The listing builds one solid part. Answer for the finished solid, in the listing's coordinates (mm). Give positions to 0.01 mm unless a question says otherwise; leave off trailing zeros. Write each loop counter-clockwise with the first axis right and the second up, starting at its lowest first coordinate (ties: lowest second). Pieces come first, ordered by that corner, then holes. Notation, with made-up numbers: (-3, 60.5) - (10, 60.5) arc R31 ccw to (10, 93.5) - close; hole circle Ø8 at (44.25, -38.5). An arc over 180 degrees is marked (long way). Answer as CSV lines item,"result". Start each with the question number.
(1) Straight lines are drawn through the part: probe 1 along X at (y, z) = (1.25, -38); probe 2 along Z at (x, y) = (10, 3.8); probe 3 along Z at (x, y) = (27.25, 2.7). For each, find the intervals that lie inside material, in ascending order.
(2) Find section A-A (x = 27.25). Write down the section's boundary in (y, z), then the cut area to 3 significant figures.
(3) Find section D-D (y = 3.5). State how many separate pieces and enclosed holes the cut face has, then the cut area to 3 significant figures.
(4) For a pull along X with two mould halves and no side action, classify faces 1 (the face through (25, 0, -51)), 2 (the face through (46.91, 2.35, -37.63)), 3 (the face through (50, 2, -49)), 4 (the face through (0, 2, -51)) as pulls with the +X half, pulls with the -X half, needs draft (parallel to the pull), parting line crosses it, or undercut.
(5) Find section B-B (z = -66.6). Write down the section's boundary in (x, y).
(6) Find section C-C (z = -38). Write down the section's boundary in (x, y).
(7) This flat-tipped pin is pushed along its axis until it touches: pin 1 Ø2 at (x, z) = (36.5, -34) entering from -Y. Where does it stop, or does it pass through?
from build123d import *

# Parameters (mm, degrees)
SKETCH1_R           = 1.7
BOSS_EXTRUDE1_DEPTH = 4.7625


with BuildPart() as part:
    # Sketch1 → Boss-Extrude1 (new body)
    with BuildSketch(Plane(origin=(0, 0, 0), x_dir=(1, 0, 0), z_dir=(0, 1, 0))):
        Polygon((0, 90), (0, 10), (20, 10), (50, 10), (50, 90), align=None)
        with Locations(Location((10, 20, 0), (0, 0, 90))):
            Circle(SKETCH1_R, mode=Mode.SUBTRACT)
        with Locations(Location((27.25, 38, 0), (0, 0, 90))):
            Circle(SKETCH1_R, mode=Mode.SUBTRACT)
        with Locations(Location((45.25, 23, 0), (0, 0, 90))):
            Circle(SKETCH1_R, mode=Mode.SUBTRACT)
        with Locations(Location((45.25, 38, 0), (0, 0, 90))):
            Circle(SKETCH1_R, mode=Mode.SUBTRACT)
        with Locations(Location((10, 70, 0), (0, 0, 90))):
            Circle(SKETCH1_R, mode=Mode.SUBTRACT)
        with Locations(Location((45.25, 66.6, 0), (0, 0, 90))):
            Circle(SKETCH1_R, mode=Mode.SUBTRACT)
        with Locations(Location((27.25, 81.6, 0), (0, 0, 90))):
            Circle(SKETCH1_R, mode=Mode.SUBTRACT)
        with Locations(Location((45.25, 81.6, 0), (0, 0, 90))):
            Circle(SKETCH1_R, mode=Mode.SUBTRACT)
    extrude(amount=BOSS_EXTRUDE1_DEPTH)


solid = part.part
Result set:
1,probe 1,"0 to 25.55, 28.95 to 43.55, 46.95 to 50"
1,probe 2,"-90 to -71.7, -68.3 to -21.7, -18.3 to -10"
1,probe 3,"-90 to -83.3, -79.9 to -39.7, -36.3 to -10"
2,outline,"(0, -90) - (4.76, -90) - (4.76, -83.3) - (0, -83.3) - close; (0, -79.9) - (4.76, -79.9) - (4.76, -39.7) - (0, -39.7) - close; (0, -36.3) - (4.76, -36.3) - (4.76, -10) - (0, -10) - close"
2,area,"349 mm^2"
3,separate pieces,"1"
3,enclosed holes,"8"
3,area,"3,930 mm^2"
4,face 1,"needs draft"
4,face 2,"undercut"
4,face 3,"pulls with the +X half"
4,face 4,"pulls with the -X half"
5,outline,"(0, 0) - (43.55, 0) - (43.55, 4.76) - (0, 4.76) - close; (46.95, 0) - (50, 0) - (50, 4.76) - (46.95, 4.76) - close"
6,outline,"(0, 0) - (25.55, 0) - (25.55, 4.76) - (0, 4.76) - close; (28.95, 0) - (43.55, 0) - (43.55, 4.76) - (28.95, 4.76) - close; (46.95, 0) - (50, 0) - (50, 4.76) - (46.95, 4.76) - close"
7,pin 1,"y = 0"
